Could you check a few things on this drawing? It's one solid part, dimensions in mm from its lowest x, y, z. Round coordinates to 2 decimals unless told otherwise and drop trailing zeros. Order: outer loops, then holes, each group sorted by start corner. A loop starts at its lowest first (then second) coordinate and runs counter-clockwise, first axis right, second up.
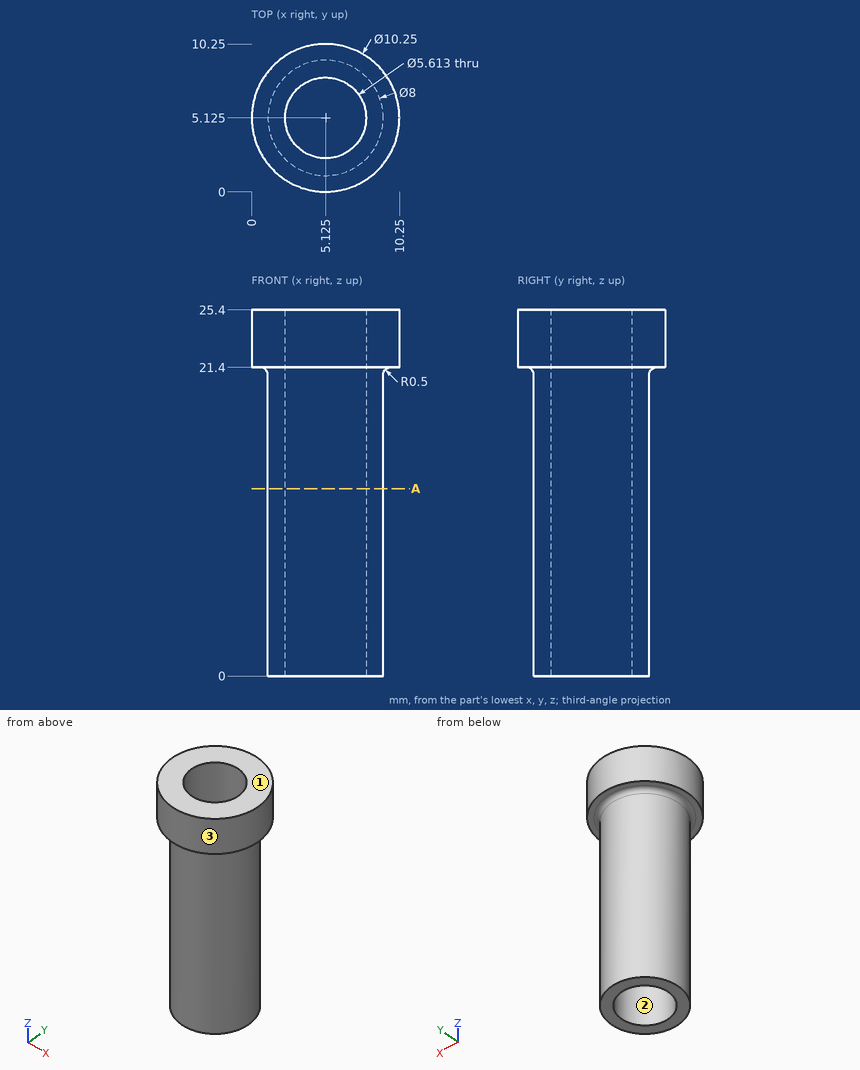
1) We'd pull the mould along Y, two halves only. Please class the marked faces 1, 2 and 3: +Y half, -Y half, draft (parallel to the pull), parting line (faces both ways), or undercut.
2) I need wall thicknesses on line 1 (Y direction, x = 5, z = 8.75); line 2 (Z direction, x = 9, y = 2.25). Which ranges of each line are inside material? Lowest first, please.
3) If we section it at A-A (z = 13): Write out the boundary of the cut face in (x, y) (1 decimal).
4) I'm going to push flat-ended pins straight in: pin 1 (3 mm diameter, centred on x = 2, z = 8, fed in from +Y); pin 2 (1.5 mm diameter, centred on x = 3, z = 21.5, fed in from -Y); pin 3 (1 mm diameter, centred on y = 3, z = 10.5, fed in from -X). Where does each tip first touch, or does it pass through?
Solutions:
1. face 1: draft
1. face 2: undercut
1. face 3: parting line
2. line 1: y = 1.13 to 2.32, 7.93 to 9.12
2. line 2: z = 21.4 to 25.4
3. outline: circle Ø8 at (5.1, 5.1); hole circle Ø5.6 at (5.1, 5.1)
4. pin 1: stops at y = 8.78
4. pin 2: stops at y = 0.19
4. pin 3: stops at x = 1.47
